The drawing under review shows one solid part. Ordinate dimensions are in mm from its lowest x, y, z. A direction names the side the tool comes from. Coordinates: 2 decimals unless noted, no trailing zeros. Write each loop counter-clockwise with the first axis right and the second up, starting at its lowest first coordinate (ties: lowest second). Pieces come first, ordered by that corner, then holes.
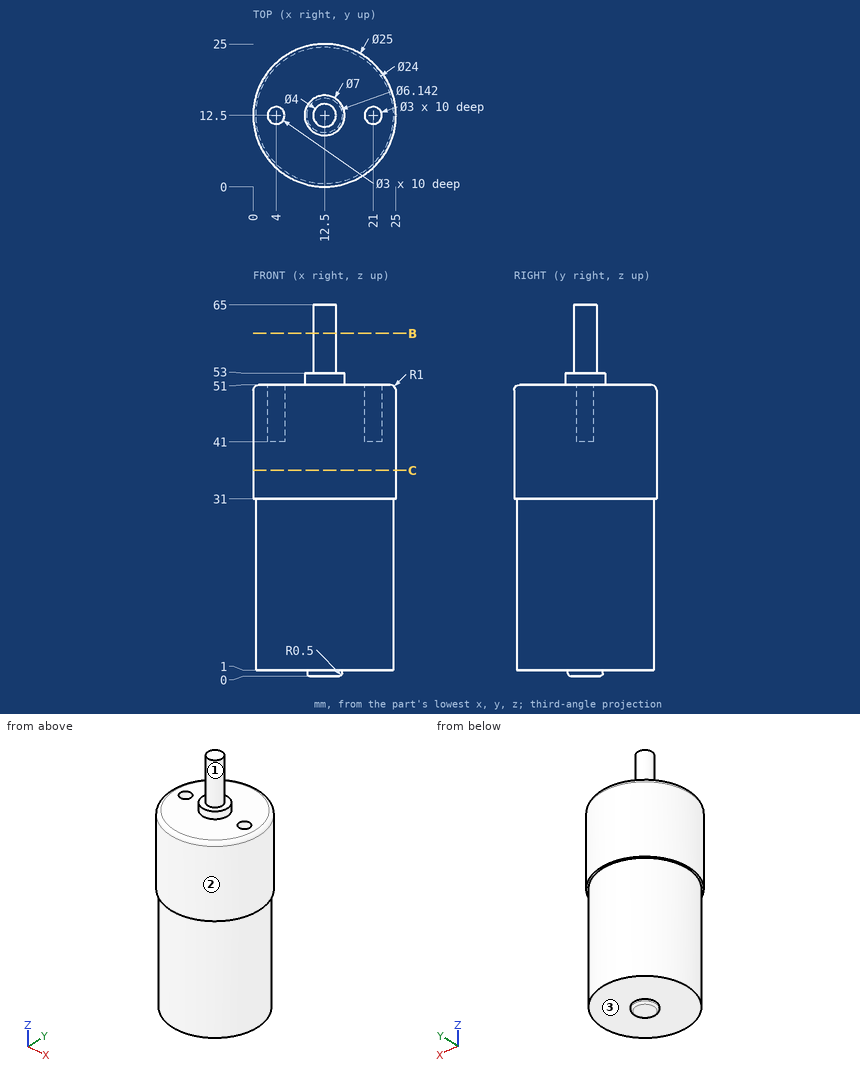
Q1. Add section C-C (z = 36). State the section outline as (x, y) points, then the cut area to 3 significant figures.
Ans:
outline: circle Ø25 at (12.5, 12.5)
area: 491 mm2
Q2. Tool access review of the marked faces 1, 2 and 3: name each direction out of +Z, -Z, +X, -X, +Y, -Y from which nothing blocks a thin tool from reaching the whole face with its end or side.
Ans:
face 1: +Z
face 2: +Z, -Z
face 3: -Z
Q3. Clearance check with flat-ended pins moving along their axes: pin 1 Ø1 at (y, z) = (10, 9.5) entering from -X; pin 2 Ø1.5 at (y, z) = (5, 37.5) entering from -X; pin 3 Ø3.5 at (x, y) = (21.5, 12.5) entering from +Z. State where each tip first meets the part, or that it passes through.
Ans:
pin 1: stops at x = 0.67
pin 2: stops at x = 1.98
pin 3: stops at z = 51
Q4. Add section B-B (z = 60). State the section outline as (x, y) points.
Ans:
outline: circle Ø4 at (12.5, 12.5)
Q5. For probe 1 along Z at (x, y) = (13, 1.5); probe 2 along Y at (x, z) = (4, 43) (1 decimal); probe 3 along X at (y, z) = (2.75, 26) (1 decimal), list the stretches that pass through material, from the lowest coordinate up.
Ans:
probe 1: z = 1 to 51
probe 2: y = 3.3 to 11, 14 to 21.7
probe 3: x = 5.5 to 19.5
